from build123d import *

# Parameters (mm, degrees)
CHAMFER1_SIZE = 0.396875
FILLET2_R     = 0.238125
CHAMFER2_SIZE = 0.79375


with BuildPart() as part:
    # Sketch3 → Revolve1 (revolve)
    with BuildSketch(Plane(origin=(0, 0, 0), x_dir=(0, 0, -1), z_dir=(1, 0, 0)), mode=Mode.PRIVATE) as revolve1_sk:
        Polygon((-9.525, 7.9375), (9.525, 7.9375), (9.525, 11.90625), (7.9375, 11.90625), (7.9375, 9.525), (-9.525, 9.525), align=None)
    revolve(revolve1_sk.sketch.rotate(Axis((0, 0, 9.525), (0, 0, -1)), 180), axis=Axis((0, 0, 9.525), (0, 0, -1)))

    # Chamfer1
    chamfer1_edges = [part.edges().sort_by_distance(p)[0] for p in [
        (0, 9.525, 9.525),
    ]]
    chamfer(chamfer1_edges, length=CHAMFER1_SIZE)

    # Fillet2
    fillet2_edges = [part.edges().sort_by_distance(p)[0] for p in [
        (0, 11.90625, -7.9375),
        (0, 11.90625, -9.525),
    ]]
    fillet(fillet2_edges, radius=FILLET2_R)

    # Chamfer2
    chamfer2_edges = [part.edges().sort_by_distance(p)[0] for p in [
        (0, 7.9375, -9.525),
    ]]
    chamfer(chamfer2_edges, length=CHAMFER2_SIZE)


solid = part.part
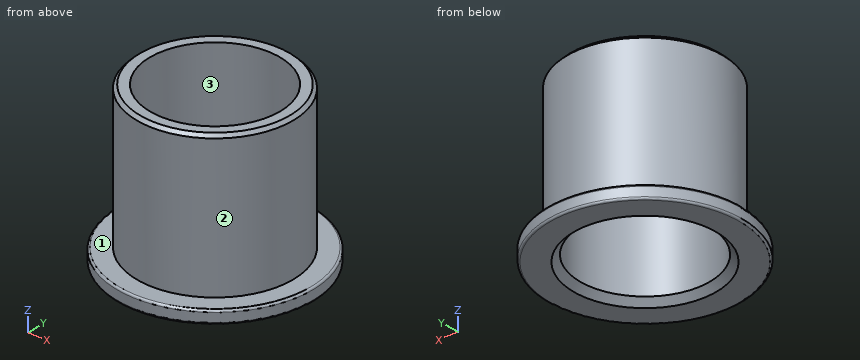
Read the model definition and answer for the solid it produces. Units are mm, in the model's axes. Face numbers are marked on the shaded views. Coordinates: 2 decimals unless noted, no trailing zeros. Answer in a Markdown table with one row per item.
Item 1: Each of these flat-tipped pins is pushed along its axis until it touches: P1, Ø10, axis at y = -4, z = -1, coming from the +X side (3 decimals); P2, Ø6, axis at x = -5.5, z = 3, coming from the -Y side; P3, Ø1, axis at x = 4, z = 6, coming from the +Y side. Where does it stop, or does it pass through?
Returned:
| item | result |
|---|---|
| P1 | stops at x = 9.525 |
| P2 | stops at y = -9.19 |
| P3 | stops at y = 8.86 |
Item 2: For a pull along Y with two mould halves and no side action, classify the marked faces 1, 2 and 3 as released by +Y, released by -Y, zero draft, split by the parting line, or undercut.
Returned:
| item | result |
|---|---|
| face 1 | zero draft |
| face 2 | split by the parting line |
| face 3 | undercut |
Item 3: Straight lines are drawn through the part: line 1 along X through (y, z) = (0, -1.25) (1 decimal); line 2 along Y through (x, z) = (-0.25, -7.5); line 3 along X through (y, z) = (-2.5, -1.5). For each, find the intervals that lie inside material, in ascending order. Write a range as [from, to].
Returned:
| item | result |
|---|---|
| line 1 | x = [-9.5, -7.9], [7.9, 9.5] |
| line 2 | y = [-9.52, -7.93], [7.93, 9.52] |
| line 3 | x = [-9.19, -7.53], [7.53, 9.19] |
